from build123d import *

# Parameters (mm, degrees)
SKETCH1_W                   = 100
SKETCH1_H                   = 50
BOSS_EXTRUDE1_DEPTH         = 12.5
SKETCH2_R                   = 8
BOSS_EXTRUDE2_DEPTH         = 10
M10X1_25_TAPPED_HOLE1_D     = 8.8
M10X1_25_TAPPED_HOLE1_DEPTH = 13
M10X1_25_TAPPED_HOLE1_TIP   = 2.643786724
M5_TAPPED_HOLE1_D           = 4.2
M5_TAPPED_HOLE1_DEPTH       = 10
M5_TAPPED_HOLE1_TIP         = 1.2618073
SKETCH8_R                   = 2.75
CUT_EXTRUDE1_DEPTH          = 23.5
SKETCH10_R                  = 5.5
CUT_EXTRUDE2_DEPTH          = 5.5


with BuildPart() as part:
    # Sketch1 → Boss-Extrude1 (new body)
    with BuildSketch(Plane(origin=(0, 0, 0), x_dir=(1, 0, 0), z_dir=(0, 1, 0))):
        Rectangle(SKETCH1_W, SKETCH1_H)
    extrude(amount=BOSS_EXTRUDE1_DEPTH)

    # Sketch2 → Boss-Extrude2 (add)
    with BuildSketch(Plane(origin=(0, 12.5, 0), x_dir=(1, 0, 0), z_dir=(0, 1, 0))):
        Circle(SKETCH2_R)
    extrude(amount=BOSS_EXTRUDE2_DEPTH)

    # M10x1.25 Tapped Hole1
    with Locations(Plane(origin=(0, 22.5, 0), x_dir=(1, 0, 0), z_dir=(0, 1, 0))):
        with Locations((0, 0)):
            Hole(M10X1_25_TAPPED_HOLE1_D / 2, depth=M10X1_25_TAPPED_HOLE1_DEPTH)
            with Locations((0, 0, -(M10X1_25_TAPPED_HOLE1_DEPTH + M10X1_25_TAPPED_HOLE1_TIP / 2))):  # 118° drill point
                Cone(0, M10X1_25_TAPPED_HOLE1_D / 2, M10X1_25_TAPPED_HOLE1_TIP, mode=Mode.SUBTRACT)

    # M5 Tapped Hole1
    with Locations(Plane(origin=(0, 12.5, 0), x_dir=(1, 0, 0), z_dir=(0, 1, 0))):
        with Locations((-35, 0), (35, 0)):
            Hole(M5_TAPPED_HOLE1_D / 2, depth=M5_TAPPED_HOLE1_DEPTH)
            with Locations((0, 0, -(M5_TAPPED_HOLE1_DEPTH + M5_TAPPED_HOLE1_TIP / 2))):  # 118° drill point
                Cone(0, M5_TAPPED_HOLE1_D / 2, M5_TAPPED_HOLE1_TIP, mode=Mode.SUBTRACT)

    # Sketch8 → Cut-Extrude1 (cut, through all)
    with BuildSketch(Plane.XZ):
        with Locations((8.3, -15)):
            Circle(SKETCH8_R)
        with Locations((-8.3, 15)):
            Circle(SKETCH8_R)
    extrude(amount=-CUT_EXTRUDE1_DEPTH, mode=Mode.SUBTRACT)

    # Sketch10 → Cut-Extrude2 (cut)
    with BuildSketch(Plane(origin=(0, 12.5, 0), x_dir=(1, 0, 0), z_dir=(0, 1, 0))):
        with Locations((8.3, 15)):
            Circle(SKETCH10_R)
        with Locations((-8.3, -15)):
            Circle(SKETCH10_R)
    extrude(amount=-CUT_EXTRUDE2_DEPTH, mode=Mode.SUBTRACT)


solid = part.part
CAD build for the part. Positions are in the model's coordinates, mm. A direction names the side the tool comes from. Round coordinates to 2 decimals unless told otherwise and drop trailing zeros. Loops run counter-clockwise (first coordinate to the right, second up) from the corner with the lowest first, then second, coordinate; pieces in that order, holes last.
(1) Wall check: line 1 along Y through (x, z) = (-28.5, 9); line 2 along Z through (x, y) = (-8.3, 8.2); line 3 along X through (y, z) = (4.25, -16.5). Give the ranges that are in metal, low to high.
(2) Cut at C-C (x = 10). Give the cut face in (y, z), plus the area to 3 significant figures.
(3) Which spindle directions (+Z, -Z, +X, -X, +Y, -Y) get a long thin tool onto all of the face, cutting with end or side? Do faces 1 (the cylindrical face through (-8.658, 3.451, 17.727)), 2 (the flat face through (9, 7, -18)). Say none if no direction does.
(4) Drop flat-ended pins along their axis: pin 1 (3.5 mm diameter, centred on x = -8.5, z = 14.5, fed in from +Y); pin 2 (12 mm diameter, centred on x = 9, z = -17, fed in from +Y); pin 3 (1.5 mm diameter, centred on x = -0.5, y = 14.5, fed in from -Z); pin 4 (3.5 mm diameter, centred on x = 35, z = 0, fed in from +Y). Give the stop position or say it passes through.
(5) Two-plate mould, pull along X, no slides. Class faces 3 (the cylindrical face through (7.11, 9.79, -9.63)), 4 (the flat face through (-1, 6, -25)), 5 (the cylindrical face through (-1.73, 17.43, 7.81)): +X half, -X half, draft (parallel to the pull), parting line (faces both ways), or undercut.
(6) Cut at A-A (y = 5.5). Give the cut face in (x, z).
(7) Cut at B-B (z = -15). Give the cut face in (x, y), plus the area to 3 significant figures.
(8) Cut at D-D (y = 19). Give the cut face in (x, z), plus the area to 3 significant figures.
Findings below:
1. line 1: y = 0 to 12.5
1. line 2: z = -25 to 9.5, 20.5 to 25
1. line 3: x = -50 to 6, 10.6 to 50
2. outline: (0, -25) - (12.5, -25) - (12.5, -20.23) - (7, -20.23) - (7, -17.16) - (0, -17.16) - close; (0, -12.84) - (7, -12.84) - (7, -9.77) - (12.5, -9.77) - (12.5, 25) - (0, 25) - close
2. area: 537 mm2
3. face 1: +Y, -Y
3. face 2: +Y
4. pin 1: passes through
4. pin 2: stops at y = 12.5
4. pin 3: stops at z = -8
4. pin 4: stops at y = 2.29
5. face 3: undercut
5. face 4: draft
5. face 5: parting line
6. outline: (-50, -25) - (50, -25) - (50, 25) - (-50, 25) - close; hole circle Ø4.2 at (-35, 0); hole circle Ø5.5 at (-8.3, 15); hole circle Ø5.5 at (8.3, -15); hole circle Ø4.2 at (35, 0)
7. outline: (-50, 0) - (5.55, 0) - (5.55, 7) - (2.8, 7) - (2.8, 12.5) - (-50, 12.5) - close; (11.05, 0) - (50, 0) - (50, 12.5) - (13.8, 12.5) - (13.8, 7) - (11.05, 7) - close
7. area: 1,150 mm2
8. outline: circle Ø16 at (0, 0); hole circle Ø8.8 at (0, 0)
8. area: 140 mm2
